Read the model definition and answer for the solid it produces. Units are mm, in the model's axes. A direction names the side the tool comes from. Coordinates: 2 decimals unless noted, no trailing zeros. Order: outer loops, then holes, each group sorted by start corner. A loop starts at its lowest first (then second) coordinate and runs counter-clockwise, first axis right, second up. Notation, with made-up numbers: M 48.5,17 L 98.5,17 A30 cw 98.5,42 Z; hole C 1,53 d4. An arc over 180 degrees is marked long. Write each question's results on one line, items separated by ' | '.
```python
from build123d import *

# Parameters (mm, degrees)
F1_DEPTH = 12.7
F2_R     = 3.175
F3_DEPTH = 25.4


with BuildPart() as f1:
    # F0 (on Front) → F1 (new body)
    with BuildSketch(Plane.XZ):
        with BuildLine():
            ThreePointArc((38.16472, -3.90239), (38.313933, -1.95373), (38.363714, 0))
            ThreePointArc((38.363714, 0), (38.318696, 1.85798), (38.183747, 3.7116))
            ThreePointArc((38.183747, 3.7116), (38.133106, 4.200094), (38.076215, 4.6879))
            ThreePointArc((38.076215, 4.6879), (37.423071, 8.443238), (36.400492, 12.115225))
            ThreePointArc((36.400492, 12.115225), (36.24242, 12.580203), (36.078408, 13.04312))
            ThreePointArc((36.078408, 13.04312), (34.606, 16.558965), (32.791965, 19.911343))
            ThreePointArc((32.791965, 19.911343), (32.534388, 20.329489), (32.27148, 20.744303))
            ThreePointArc((32.27148, 20.744303), (30.053638, 23.844357), (27.539111, 26.709023))
            ThreePointArc((27.539111, 26.709023), (27.194947, 27.059368), (26.846325, 27.40528))
            ThreePointArc((26.846325, 27.40528), (23.994262, 29.934093), (20.905332, 32.1674))
            ThreePointArc((20.905332, 32.1674), (20.491837, 32.432378), (20.074983, 32.692041))
            ThreePointArc((20.074983, 32.692041), (16.731714, 34.522808), (13.223271, 36.01277))
            ThreePointArc((13.223271, 36.01277), (12.76118, 36.179094), (12.296998, 36.339488))
            ThreePointArc((12.296998, 36.339488), (8.630167, 37.380406), (4.878141, 38.05231))
            ThreePointArc((4.878141, 38.05231), (4.390625, 38.111638), (3.90239, 38.16472))
            ThreePointArc((3.90239, 38.16472), (0.095868, 38.363594), (-3.7116, 38.183747))
            ThreePointArc((-3.7116, 38.183747), (-4.200094, 38.133106), (-4.6879, 38.076215))
            ThreePointArc((-4.6879, 38.076215), (-8.443238, 37.423071), (-12.115225, 36.400492))
            ThreePointArc((-12.115225, 36.400492), (-12.580203, 36.24242), (-13.04312, 36.078408))
            ThreePointArc((-13.04312, 36.078408), (-16.558965, 34.606), (-19.911343, 32.791965))
            ThreePointArc((-19.911343, 32.791965), (-20.329489, 32.534388), (-20.744303, 32.27148))
            ThreePointArc((-20.744303, 32.27148), (-23.844357, 30.053638), (-26.709023, 27.539111))
            ThreePointArc((-26.709023, 27.539111), (-27.059368, 27.194947), (-27.40528, 26.846325))
            ThreePointArc((-27.40528, 26.846325), (-29.934093, 23.994262), (-32.1674, 20.905332))
            ThreePointArc((-32.1674, 20.905332), (-32.432378, 20.491837), (-32.692041, 20.074983))
            ThreePointArc((-32.692041, 20.074983), (-34.522808, 16.731714), (-36.01277, 13.223271))
            ThreePointArc((-36.01277, 13.223271), (-36.179094, 12.76118), (-36.339488, 12.296998))
            ThreePointArc((-36.339488, 12.296998), (-37.380406, 8.630167), (-38.05231, 4.878141))
            ThreePointArc((-38.05231, 4.878141), (-38.111638, 4.390625), (-38.16472, 3.90239))
            ThreePointArc((-38.16472, 3.90239), (-38.363594, 0.095868), (-38.183747, -3.7116))
            ThreePointArc((-38.183747, -3.7116), (-38.133106, -4.200094), (-38.076215, -4.6879))
            ThreePointArc((-38.076215, -4.6879), (-37.423071, -8.443238), (-36.400492, -12.115225))
            ThreePointArc((-36.400492, -12.115225), (-36.24242, -12.580203), (-36.078408, -13.04312))
            ThreePointArc((-36.078408, -13.04312), (-34.606, -16.558965), (-32.791965, -19.911343))
            ThreePointArc((-32.791965, -19.911343), (-32.534388, -20.329489), (-32.27148, -20.744303))
            ThreePointArc((-32.27148, -20.744303), (-30.053638, -23.844357), (-27.539111, -26.709023))
            ThreePointArc((-27.539111, -26.709023), (-27.194947, -27.059368), (-26.846325, -27.40528))
            ThreePointArc((-26.846325, -27.40528), (-23.994262, -29.934093), (-20.905332, -32.1674))
            ThreePointArc((-20.905332, -32.1674), (-20.491837, -32.432378), (-20.074983, -32.692041))
            ThreePointArc((-20.074983, -32.692041), (-16.731714, -34.522808), (-13.223271, -36.01277))
            ThreePointArc((-13.223271, -36.01277), (-12.76118, -36.179094), (-12.296998, -36.339488))
            ThreePointArc((-12.296998, -36.339488), (-8.630167, -37.380406), (-4.878141, -38.05231))
            ThreePointArc((-4.878141, -38.05231), (-4.390625, -38.111638), (-3.90239, -38.16472))
            ThreePointArc((-3.90239, -38.16472), (-0.095868, -38.363594), (3.7116, -38.183747))
            ThreePointArc((3.7116, -38.183747), (4.200094, -38.133106), (4.6879, -38.076215))
            ThreePointArc((4.6879, -38.076215), (8.443238, -37.423071), (12.115225, -36.400492))
            ThreePointArc((12.115225, -36.400492), (12.580203, -36.24242), (13.04312, -36.078408))
            ThreePointArc((13.04312, -36.078408), (16.558965, -34.606), (19.911343, -32.791965))
            ThreePointArc((19.911343, -32.791965), (20.329489, -32.534388), (20.744303, -32.27148))
            ThreePointArc((20.744303, -32.27148), (23.844357, -30.053638), (26.709023, -27.539111))
            ThreePointArc((26.709023, -27.539111), (27.059368, -27.194947), (27.40528, -26.846325))
            ThreePointArc((27.40528, -26.846325), (29.934093, -23.994262), (32.1674, -20.905332))
            ThreePointArc((32.1674, -20.905332), (32.432378, -20.491837), (32.692041, -20.074983))
            ThreePointArc((32.692041, -20.074983), (34.522808, -16.731714), (36.01277, -13.223271))
            ThreePointArc((36.01277, -13.223271), (36.179094, -12.76118), (36.339488, -12.296998))
            ThreePointArc((36.339488, -12.296998), (37.380406, -8.630167), (38.05231, -4.878141))
            ThreePointArc((38.05231, -4.878141), (38.111638, -4.390625), (38.16472, -3.90239))
        make_face()
        with BuildLine():
            ThreePointArc((38.183747, 3.7116), (38.318696, 1.85798), (38.363714, 0))
            ThreePointArc((38.363714, 0), (38.313933, -1.95373), (38.16472, -3.90239))
            Line((38.16472, -3.90239), (45.522928, 0))
            Line((45.522928, 0), (38.183747, 3.7116))
        make_face()
        with BuildLine():
            ThreePointArc((36.400492, 12.115225), (37.423071, 8.443238), (38.076215, 4.6879))
            Line((38.076215, 4.6879), (44.381573, 10.129805))
            Line((44.381573, 10.129805), (36.400492, 12.115225))
        make_face()
        with BuildLine():
            Line((44.381573, -10.129805), (38.05231, -4.878141))
            ThreePointArc((38.05231, -4.878141), (37.380406, -8.630167), (36.339488, -12.296998))
            Line((36.339488, -12.296998), (44.381573, -10.129805))
        make_face()
        with BuildLine():
            ThreePointArc((32.791965, 19.911343), (34.606, 16.558965), (36.078408, 13.04312))
            Line((36.078408, 13.04312), (41.014741, 19.751658))
            Line((41.014741, 19.751658), (32.791965, 19.911343))
        make_face()
        with BuildLine():
            Line((41.014741, -19.751658), (36.01277, -13.223271))
            ThreePointArc((36.01277, -13.223271), (34.522808, -16.731714), (32.692041, -20.074983))
            Line((32.692041, -20.074983), (41.014741, -19.751658))
        make_face()
        with BuildLine():
            ThreePointArc((27.539111, 26.709023), (30.053638, 23.844357), (32.27148, 20.744303))
            Line((32.27148, 20.744303), (35.591258, 28.383082))
            Line((35.591258, 28.383082), (27.539111, 26.709023))
        make_face()
        with BuildLine():
            Line((35.591258, -28.383082), (32.1674, -20.905332))
            ThreePointArc((32.1674, -20.905332), (29.934093, -23.994262), (27.40528, -26.846325))
            Line((27.40528, -26.846325), (35.591258, -28.383082))
        make_face()
        with BuildLine():
            ThreePointArc((20.905332, 32.1674), (23.994262, 29.934093), (26.846325, 27.40528))
            Line((26.846325, 27.40528), (28.383082, 35.591258))
            Line((28.383082, 35.591258), (20.905332, 32.1674))
        make_face()
        with BuildLine():
            Line((28.383082, -35.591258), (26.709023, -27.539111))
            ThreePointArc((26.709023, -27.539111), (23.844357, -30.053638), (20.744303, -32.27148))
            Line((20.744303, -32.27148), (28.383082, -35.591258))
        make_face()
        with BuildLine():
            ThreePointArc((13.223271, 36.01277), (16.731714, 34.522808), (20.074983, 32.692041))
            Line((20.074983, 32.692041), (19.751658, 41.014741))
            Line((19.751658, 41.014741), (13.223271, 36.01277))
        make_face()
        with BuildLine():
            Line((19.751658, -41.014741), (19.911343, -32.791965))
            ThreePointArc((19.911343, -32.791965), (16.558965, -34.606), (13.04312, -36.078408))
            Line((13.04312, -36.078408), (19.751658, -41.014741))
        make_face()
        with BuildLine():
            ThreePointArc((4.878141, 38.05231), (8.630167, 37.380406), (12.296998, 36.339488))
            Line((12.296998, 36.339488), (10.129805, 44.381573))
            Line((10.129805, 44.381573), (4.878141, 38.05231))
        make_face()
        with BuildLine():
            Line((10.129805, -44.381573), (12.115225, -36.400492))
            ThreePointArc((12.115225, -36.400492), (8.443238, -37.423071), (4.6879, -38.076215))
            Line((4.6879, -38.076215), (10.129805, -44.381573))
        make_face()
        with BuildLine():
            ThreePointArc((-3.7116, 38.183747), (0.095868, 38.363594), (3.90239, 38.16472))
            Line((3.90239, 38.16472), (0, 45.522928))
            Line((0, 45.522928), (-3.7116, 38.183747))
        make_face()
        with BuildLine():
            Line((0, -45.522928), (3.7116, -38.183747))
            ThreePointArc((3.7116, -38.183747), (-0.095868, -38.363594), (-3.90239, -38.16472))
            Line((-3.90239, -38.16472), (0, -45.522928))
        make_face()
        with BuildLine():
            ThreePointArc((-12.115225, 36.400492), (-8.443238, 37.423071), (-4.6879, 38.076215))
            Line((-4.6879, 38.076215), (-10.129805, 44.381573))
            Line((-10.129805, 44.381573), (-12.115225, 36.400492))
        make_face()
        with BuildLine():
            Line((-10.129805, -44.381573), (-4.878141, -38.05231))
            ThreePointArc((-4.878141, -38.05231), (-8.630167, -37.380406), (-12.296998, -36.339488))
            Line((-12.296998, -36.339488), (-10.129805, -44.381573))
        make_face()
        with BuildLine():
            ThreePointArc((-19.911343, 32.791965), (-16.558965, 34.606), (-13.04312, 36.078408))
            Line((-13.04312, 36.078408), (-19.751658, 41.014741))
            Line((-19.751658, 41.014741), (-19.911343, 32.791965))
        make_face()
        with BuildLine():
            Line((-19.751658, -41.014741), (-13.223271, -36.01277))
            ThreePointArc((-13.223271, -36.01277), (-16.731714, -34.522808), (-20.074983, -32.692041))
            Line((-20.074983, -32.692041), (-19.751658, -41.014741))
        make_face()
        with BuildLine():
            ThreePointArc((-26.709023, 27.539111), (-23.844357, 30.053638), (-20.744303, 32.27148))
            Line((-20.744303, 32.27148), (-28.383082, 35.591258))
            Line((-28.383082, 35.591258), (-26.709023, 27.539111))
        make_face()
        with BuildLine():
            Line((-28.383082, -35.591258), (-20.905332, -32.1674))
            ThreePointArc((-20.905332, -32.1674), (-23.994262, -29.934093), (-26.846325, -27.40528))
            Line((-26.846325, -27.40528), (-28.383082, -35.591258))
        make_face()
        with BuildLine():
            ThreePointArc((-32.1674, 20.905332), (-29.934093, 23.994262), (-27.40528, 26.846325))
            Line((-27.40528, 26.846325), (-35.591258, 28.383082))
            Line((-35.591258, 28.383082), (-32.1674, 20.905332))
        make_face()
        with BuildLine():
            Line((-35.591258, -28.383082), (-27.539111, -26.709023))
            ThreePointArc((-27.539111, -26.709023), (-30.053638, -23.844357), (-32.27148, -20.744303))
            Line((-32.27148, -20.744303), (-35.591258, -28.383082))
        make_face()
        with BuildLine():
            ThreePointArc((-36.01277, 13.223271), (-34.522808, 16.731714), (-32.692041, 20.074983))
            Line((-32.692041, 20.074983), (-41.014741, 19.751658))
            Line((-41.014741, 19.751658), (-36.01277, 13.223271))
        make_face()
        with BuildLine():
            Line((-41.014741, -19.751658), (-32.791965, -19.911343))
            ThreePointArc((-32.791965, -19.911343), (-34.606, -16.558965), (-36.078408, -13.04312))
            Line((-36.078408, -13.04312), (-41.014741, -19.751658))
        make_face()
        with BuildLine():
            ThreePointArc((-38.05231, 4.878141), (-37.380406, 8.630167), (-36.339488, 12.296998))
            Line((-36.339488, 12.296998), (-44.381573, 10.129805))
            Line((-44.381573, 10.129805), (-38.05231, 4.878141))
        make_face()
        with BuildLine():
            Line((-44.381573, -10.129805), (-36.400492, -12.115225))
            ThreePointArc((-36.400492, -12.115225), (-37.423071, -8.443238), (-38.076215, -4.6879))
            Line((-38.076215, -4.6879), (-44.381573, -10.129805))
        make_face()
        with BuildLine():
            ThreePointArc((-38.183747, -3.7116), (-38.363594, 0.095868), (-38.16472, 3.90239))
            Line((-38.16472, 3.90239), (-45.522928, 0))
            Line((-45.522928, 0), (-38.183747, -3.7116))
        make_face()
    extrude(amount=F1_DEPTH)

    # F2 (on face) → F3 (cut)
    with BuildSketch(Plane.XZ.offset(12.7)):
        Circle(F2_R)
    extrude(amount=-F3_DEPTH, mode=Mode.SUBTRACT)


solid = f1.part
```
(1) The part is cut by section A-A, the plane x = -6.5. Write down the section's boundary in (y, z).
Conclusion:
outline: M -12.7,-40.01 L 0,-40.01 L 0,40.18 L -12.7,40.18 Z
(2) The mould has two halves that part along X. Classify faces 1 (the flat face through (-41.26, -6.26, 7.54)), 2 (the flat face through (-24.51, -6.26, 33.91)), 3 (the flat face through (40.3, -6.26, -11.23)): pulls with the +X half, pulls with the -X half, needs draft (parallel to the pull), parting line crosses it, or undercut.
Conclusion:
face 1: pulls with the -X half | face 2: undercut | face 3: pulls with the +X half
(3) Given pin 1 (1.5 mm diameter, centred on y = -8, z = -34, fed in from +X); pin 2 (4 mm diameter, centred on y = -10, z = -23, fed in from -X), each flat-ended and moving along its own axis, determine where each tip first touches the part or whether it passes through.
Conclusion:
pin 1: x = 28.21 | pin 2: x = -34.12
(4) Straight lines are drawn through the part: line 1 (Z direction, x = -38, y = -10.5); line 2 (X direction, y = -1, z = 40.5); line 3 (X direction, y = -9.75, z = 32.5). For each, find the intervals that lie inside material, in ascending order.
Conclusion:
line 1: -19.81 to -15.65, -11.72 to 11.85, 15.82 to 19.87 | line 2: -19.76 to -19.05, -11.1 to -6.78, -2.54 to 2.66, 6.91 to 11.18, 19.08 to 19.77 | line 3: -27.74 to -21.27, -20.38 to 20.38, 21.63 to 27.8
(5) The part is cut by section B-B, the plane x = 15. Write down the section's boundary in (y, z), then the cut area to 3 significant figures.
Conclusion:
outline: M -12.7,-37.52 L 0,-37.52 L 0,37.37 L -12.7,37.37 Z | area: 951 mm²
(6) For faces 4 (the flat face through (11.23, -6.26, 40.3)), 5 (the flat face through (-24.697, -6.261, -33.903)), 6 (the flat face through (-38.51, -6.26, -16.35)), determine the directions among +Z, -Z, +X, -X, +Y, -Y from which every point of the face is accessible in a straight line to the end or side of a thin tool.
Conclusion:
face 4: +Z, +Y, -Y | face 5: -Z, +Y, -Y | face 6: -X, +Y, -Y
